Geometry: final body of the model. Coordinates: model frame, mm. Face numbers are marked on the shaded views. A direction names the side the tool comes from. Give positions to 0.01 mm unless a question says otherwise; leave off trailing zeros. Order: outer loops, then holes, each group sorted by start corner. A loop starts at its lowest first (then second) coordinate and runs counter-clockwise, first axis right, second up. Notation, with made-up numbers: (27, 64) -> (75, 64) arc R10 cw to (75, 72) -> close; hole circle Ø5 at (71, 87.25). An arc over 180 degrees is marked (long way). Answer in a Markdown table with one row per item. Add a question column.
Q1. Cut plane A-A on z = 11. Return the cut outline in (x, y).
Q2. Set-up query: the marked faces 1 and 2. Return all of +Z, -Z, +X, -X, +Y, -Y with unobstructed straight access to the full face (end or side cutting, diameter ignored); none if empty.
Q3. Cut plane C-C on y = 0. Return the cut outline in (x, z).
Q4. Line query: line 1 along Z through (x, y) = (1.3, 0); line 2 along Y through (x, z) = (8.5, 0.55); line 3 along X through (y, z) = (-2.5, 7). Output: solid intervals per line, ascending. Write a range as from..to.
Q5. Contact query for flat-ended pins moving along their axis: P1, Ø6, axis at y = 1, z = 13.5, coming from the -X side; P2, Ø6.5, axis at x = 9.5, y = -2.5, coming from the +Z side; P3, Ø12, axis at y = 7.5, z = 12, coming from the +X side. Output: stop coordinate, or through.
Q6. Cut plane D-D on y = 8. Return the cut outline in (x, z), and give its area (3 significant figures).
Q7. Cut plane B-B on x = 8.5. Return the cut outline in (y, z).
from build123d import *

# Parameters (mm, degrees)
F1_DEPTH   = 10
F4_D       = 3.3
F4_ON_F3_D = 3.3


with BuildPart() as f1:
    # F0 (on Front) → F1 (new body, symmetric)
    with BuildSketch(Plane.XZ):
        Polygon((0, 20), (0, 0), (15, 0), (15, 2), (2, 2), (2, 20), align=None)
    extrude(amount=F1_DEPTH, both=True)

    # F4 (through all)
    with Locations(Plane(origin=(0, 0, 0), x_dir=(0, -1, 0), z_dir=(-1, 0, 0))):
        with Locations((0, 11)):
            Hole(F4_D / 2)

    # F4 on F3 (through all)
    with Locations(Plane.XY.offset(2)):
        with Locations((8.5, 0)):
            Hole(F4_ON_F3_D / 2)


solid = f1.part
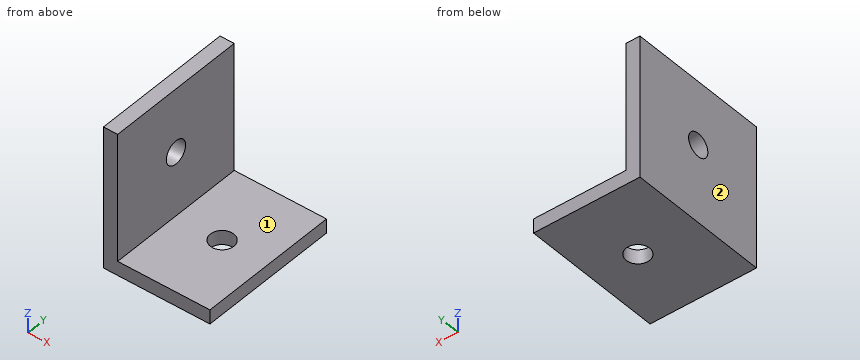
Completed:
| question | item | result |
|---|---|---|
| 1 | outline | (0, -10) -> (2, -10) -> (2, -1.65) -> (0, -1.65) -> close; (0, 1.65) -> (2, 1.65) -> (2, 10) -> (0, 10) -> close |
| 2 | face 1 | +Z, +X, +Y, -Y |
| 2 | face 2 | +Z, -Z, -X, +Y, -Y |
| 3 | outline | (0, 0) -> (6.85, 0) -> (6.85, 2) -> (2, 2) -> (2, 9.35) -> (0, 9.35) -> close; (0, 12.65) -> (2, 12.65) -> (2, 20) -> (0, 20) -> close; (10.15, 0) -> (15, 0) -> (15, 2) -> (10.15, 2) -> close |
| 4 | line 1 | z = 0..9.35, 12.65..20 |
| 4 | line 2 | y = -10..-1.65, 1.65..10 |
| 4 | line 3 | x = 0..2 |
| 5 | P1 | stops at x = 0 |
| 5 | P2 | stops at z = 2 |
| 5 | P3 | stops at x = 2 |
| 6 | outline | (0, 0) -> (15, 0) -> (15, 2) -> (2, 2) -> (2, 20) -> (0, 20) -> close |
| 6 | area | 66.0 mm² |
| 7 | outline | (-10, 0) -> (-1.65, 0) -> (-1.65, 2) -> (-10, 2) -> close; (1.65, 0) -> (10, 0) -> (10, 2) -> (1.65, 2) -> close |
